```python
from build123d import *

# Parameters (mm, degrees)
SKETCH_1_W          = 10
SKETCH_1_H          = 15.4
EXTRUDE_1_DEPTH     = 4.5
SKETCH_2_W          = 10
SKETCH_2_H          = 6.5
CUT_EXTRUDE_1_DEPTH = 3.3
CHAMFER_1_SIZE      = 2
CUT_EXTRUDE_2_DEPTH = 10
SKETCH_4_W          = 0.965597518
SKETCH_4_H          = 0.5
EXTRUDE_2_DEPTH     = 8


with BuildPart() as part:
    # 草图1 → 凸台-拉伸1 (new body)
    with BuildSketch(Plane.XY):
        with Locations((0, 7.7)):
            Rectangle(SKETCH_1_W, SKETCH_1_H)
    extrude(amount=EXTRUDE_1_DEPTH)

    # 草图2 → 切除-拉伸1 (cut)
    with BuildSketch(Plane.XY.offset(4.5)):
        with Locations((0, 12.15)):
            Rectangle(SKETCH_2_W, SKETCH_2_H)
    extrude(amount=-CUT_EXTRUDE_1_DEPTH, mode=Mode.SUBTRACT)

    # 倒角1
    chamfer_1_edges = [part.edges().sort_by_distance(p)[0] for p in [
        (0, 8.9, 4.5),
    ]]
    chamfer(chamfer_1_edges, length=CHAMFER_1_SIZE)

    # 草图5 → 切除-拉伸2 (cut)
    with BuildSketch(Plane.XY.offset(1.2)):
        Polygon((-5, 9.069569731), (-2.668025146, 9.645356545), (2.668025146, 9.645356545), (5, 9.069569731), (5, 15.4), (-5, 15.4), align=None)
    extrude(amount=-CUT_EXTRUDE_2_DEPTH, mode=Mode.SUBTRACT)

    # 草图4 → 凸台-拉伸2 (add)
    with BuildSketch(Plane.XZ):
        with Locations((1.27, 3.23)):
            Rectangle(SKETCH_4_W, SKETCH_4_H)
        with Locations((0, 3.23)):
            Rectangle(SKETCH_4_W, SKETCH_4_H)
        with Locations((-1.27, 3.23)):
            Rectangle(SKETCH_4_W, SKETCH_4_H)
        with Locations((-2.54, 3.23)):
            Rectangle(SKETCH_4_W, SKETCH_4_H)
        with Locations((2.54, 3.23)):
            Rectangle(SKETCH_4_W, SKETCH_4_H)
    extrude(amount=EXTRUDE_2_DEPTH)


solid = part.part
```
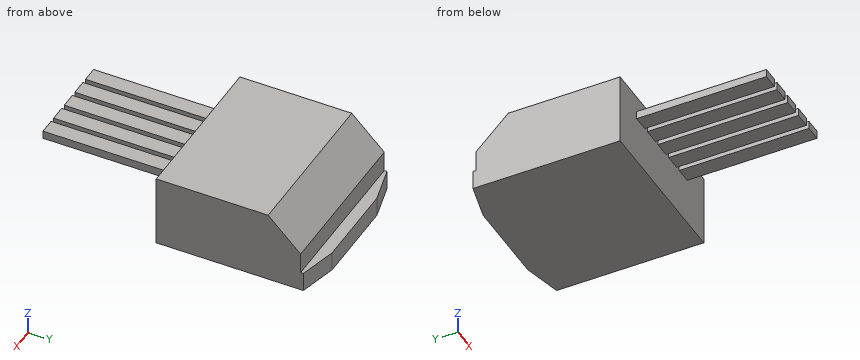
Can you work these out from the model? Positions are in its coordinate system, mm. Round coordinates to 2 decimals unless told otherwise and drop trailing zeros. Loops run counter-clockwise (first coordinate to the right, second up) from the corner with the lowest first, then second, coordinate; pieces in that order, holes last.
Item 1: Suppose I cut it at D-D, the plane y = 8. Write out the boundary of the cut face in (x, z), then the cut area to 3 significant figures.
Item 2: Suppose I cut it at B-B, the plane z = 0.8. Write out the boundary of the cut face in (x, y), then the cut area to 3 significant figures.
Item 3: Please list where these lines run through material, in increasing order: L1, parallel to Z at x = 1.5, y = -5.25; L2, parallel to Y at x = 3.25, z = 2.2; L3, parallel to Y at x = 1, z = 0.85.
Item 4: Suppose I cut it at C-C, the plane x = -4. Write out the boundary of the cut face in (y, z), then the cut area to 3 significant figures.
Item 5: Suppose I cut it at A-A, the plane y = -5.5. Write out the boundary of the cut face in (x, z), then the cut area to 3 significant figures.
Item 6: Will these pins go through, and if not, where does the flat tip stop? pin 1 Ø0.5 at (x, y) = (2.5, -2.5) entering from -Z; pin 2 Ø1.5 at (x, z) = (1, 1.5) entering from +Y; pin 3 Ø0.6 at (y, z) = (-4.5, 3) entering from -X; pin 4 Ø0.6 at (y, z) = (-5.5, 3) entering from +X.
Reported:
1. outline: (-5, 0) - (5, 0) - (5, 3.4) - (-5, 3.4) - close
1. area: 34.0 mm2
2. outline: (-5, 0) - (5, 0) - (5, 9.07) - (2.67, 9.65) - (-2.67, 9.65) - (-5, 9.07) - close
2. area: 95.1 mm2
3. L1: z = 2.98 to 3.48
3. L2: y = 0 to 8.9
3. L3: y = 0 to 9.65
4. outline: (0, 0) - (9.32, 0) - (9.32, 1.2) - (8.9, 1.2) - (8.9, 2.5) - (6.9, 4.5) - (0, 4.5) - close
4. area: 38.5 mm2
5. outline: (-3.02, 2.98) - (-2.06, 2.98) - (-2.06, 3.48) - (-3.02, 3.48) - close; (-1.75, 2.98) - (-0.79, 2.98) - (-0.79, 3.48) - (-1.75, 3.48) - close; (-0.48, 2.98) - (0.48, 2.98) - (0.48, 3.48) - (-0.48, 3.48) - close; (0.79, 2.98) - (1.75, 2.98) - (1.75, 3.48) - (0.79, 3.48) - close; (2.06, 2.98) - (3.02, 2.98) - (3.02, 3.48) - (2.06, 3.48) - close
5. area: 2.41 mm2
6. pin 1: stops at z = 2.98
6. pin 2: stops at y = 9.65
6. pin 3: stops at x = -3.02
6. pin 4: stops at x = 3.02
